Read the model definition and answer for the solid it produces. Units are mm, in the model's axes. A direction names the side the tool comes from. Coordinates: 2 decimals unless noted, no trailing zeros. Write each loop counter-clockwise with the first axis right and the second up, starting at its lowest first coordinate (ties: lowest second). Pieces come first, ordered by that corner, then holes. Notation, with made-up numbers: (87, 49.25) -> (104, 49.25) arc R28 ccw to (104, 84.25) -> close; hole circle Ø9 at (-17.5, 30). An arc over 180 degrees is marked (long way). Use CSV: the item, a comma, the result in double quotes.
from build123d import *

# Parameters (mm, degrees)
SKETCH_1_R      = 1
EXTRUDE_1_DEPTH = 2
SKETCH_2_R      = 1.5
SKETCH_2_R_2    = 1
EXTRUDE_2_DEPTH = 0.5
SKETCH_3_R      = 0.7
EXTRUDE_3_DEPTH = 5
EXTRUDE_START   = -2
SKETCH_4_R      = 1
EXTRUDE_4_DEPTH = 0.1


with BuildPart() as part:
    # 草图1 → 凸台-拉伸1 (new body)
    with BuildSketch(Plane.XY):
        with BuildLine():
            Line((0, -1.5), (-12, -1.5))
            ThreePointArc((-12, -1.5), (-13.5, 0), (-12, 1.5))
            Line((-12, 1.5), (0, 1.5))
            ThreePointArc((0, 1.5), (1.5, 0), (0, -1.5))
        make_face()
        with Locations((-12, 0)):
            Circle(SKETCH_1_R, mode=Mode.SUBTRACT)
        Circle(SKETCH_1_R, mode=Mode.SUBTRACT)
    extrude(amount=EXTRUDE_1_DEPTH)

    # 草图2 → 凸台-拉伸2 (add)
    with BuildSketch(Plane.XY):
        Circle(SKETCH_2_R)
        Circle(SKETCH_2_R_2, mode=Mode.SUBTRACT)
    extrude(amount=-EXTRUDE_2_DEPTH)

    # 草图3 → 凸台-拉伸3 (add)
    with BuildSketch(Plane.XY.offset(2)):
        with Locations((-3.8, 0)):
            Circle(SKETCH_3_R)
    extrude(amount=EXTRUDE_3_DEPTH)

    # 草图4 → 凸台-拉伸4 (add)
    with BuildSketch(Plane.XY.offset(7).offset(EXTRUDE_START)):
        with Locations((-3.8, 0)):
            Circle(SKETCH_4_R)
    extrude(amount=-EXTRUDE_4_DEPTH)


solid = part.part
1. This flat-tipped pin is pushed along its axis until it touches: pin 1 Ø1 at (x, y) = (-7.5, -1) entering from +Z. Where does it stop, or does it pass through?
Solutions:
pin 1,"stops at z = 2"
2. Find the intervals of material crossed by line 1 along Y through (x, z) = (-12, 0.8); line 2 along X through (y, z) = (-0.7, 1.25); line 3 along X through (y, z) = (-0.2, 0.75), in increasing order.
Solutions:
line 1,"y = -1.5 to -1, 1 to 1.5"
line 2,"x = -13.33 to -12.71, -11.29 to -0.71, 0.71 to 1.33"
line 3,"x = -13.49 to -12.98, -11.02 to -0.98, 0.98 to 1.49"
3. A cutting plane is placed at B-B (z = 0.5). Give the vertices of the cut face in (x, y), and give its area (3 significant figures).
Solutions:
outline,"(-12, -1.5) -> (0, -1.5) arc R1.5 ccw to (0, 1.5) -> (-12, 1.5) arc R1.5 ccw to start; hole circle Ø2 at (-12, 0); hole circle Ø2 at (0, 0)"
area,"36.8 mm^2"
4. A cutting plane is placed at D-D (z = 6). Give the vertices of the cut face in (x, y), and give its area (3 significant figures).
Solutions:
outline,"circle Ø1.4 at (-3.8, 0)"
area,"1.54 mm^2"
5. A cutting plane is placed at C-C (x = -3.8). Give the vertices of the cut face in (y, z), and give its area (3 significant figures).
Solutions:
outline,"(-1.5, 0) -> (1.5, 0) -> (1.5, 2) -> (0.7, 2) -> (0.7, 4.9) -> (1, 4.9) -> (1, 5) -> (0.7, 5) -> (0.7, 7) -> (-0.7, 7) -> (-0.7, 5) -> (-1, 5) -> (-1, 4.9) -> (-0.7, 4.9) -> (-0.7, 2) -> (-1.5, 2) -> close"
area,"13.1 mm^2"
6. A tool of negligible diameter and unlimited length cuts with its end or side. For faces 5 (the flat face through (-4, 0, 7)), 6 (the cylindrical face through (-4.5, 0, 3.4)), 7 (the cylindrical face through (-4.5, 0, 6)), from which of +Z, -Z, +X, -X, +Y, -Y can it reach the whole face along a straight path? Write none if from no direction.
Solutions:
face 5,"+Z, +X, -X, +Y, -Y"
face 6,"none"
face 7,"+Z"
7. For a pull along Y with two mould halves and no side action, classify faces 1 (the flat face through (-7, 0, 0)), 2 (the cylindrical face through (0, -1, 1)), 3 (the cylindrical face through (-13.5, 0, 1)), 4 (the flat face through (-6, 1.5, 1)) as pulls with the +Y half, pulls with the -Y half, needs draft (parallel to the pull), parting line crosses it, or undercut.
Solutions:
face 1,"needs draft"
face 2,"undercut"
face 3,"parting line crosses it"
face 4,"pulls with the +Y half"
8. A cutting plane is placed at A-A (y = 0). Give the vertices of the cut face in (x, z).
Solutions:
outline,"(-13.5, 0) -> (-13, 0) -> (-13, 2) -> (-13.5, 2) -> close; (-11, 0) -> (-1.5, 0) -> (-1.5, -0.5) -> (-1, -0.5) -> (-1, 2) -> (-3.1, 2) -> (-3.1, 4.9) -> (-2.8, 4.9) -> (-2.8, 5) -> (-3.1, 5) -> (-3.1, 7) -> (-4.5, 7) -> (-4.5, 5) -> (-4.8, 5) -> (-4.8, 4.9) -> (-4.5, 4.9) -> (-4.5, 2) -> (-11, 2) -> close; (1, -0.5) -> (1.5, -0.5) -> (1.5, 2) -> (1, 2) -> close"
